from build123d import *

# Parameters (mm, degrees)
SKETCH_R        = 4
PAD_DEPTH       = 6.91
CHAMFER_SIZE    = 0.9674
CHAMFER001_SIZE = 0.9674
GROOVE_ANGLE    = -360


with BuildPart() as part:
    # Sketch → Pad (new body)
    with BuildSketch(Plane.XY):
        Polygon((0, 7), (-6.062178, 3.5), (-6.062178, -3.5), (0, -7), (6.062178, -3.5), (6.062178, 3.5), align=None)
        Circle(SKETCH_R, mode=Mode.SUBTRACT)
    extrude(amount=PAD_DEPTH)

    # Chamfer
    chamfer_edges = [part.edges().sort_by_distance(p)[0] for p in [
        (-4, 0, 6.91),
    ]]
    chamfer(chamfer_edges, length=CHAMFER_SIZE)

    # Chamfer001
    chamfer001_edges = [part.edges().sort_by_distance(p)[0] for p in [
        (-4, 0, 0),
    ]]
    chamfer(chamfer001_edges, length=CHAMFER001_SIZE)

    # Sketch001 → Groove (revolve, symmetric, cut)
    with BuildSketch(Plane.YZ) as groove_sk:
        Polygon((-6.062178, 6.91), (-7, 6.91), (-7, 5.285644), align=None)
        Polygon((-7, 1.624356), (-7, 0), (-6.062178, 0), align=None)
    revolve(axis=Axis((0, 0, 0), (0, 0, 1)), revolution_arc=GROOVE_ANGLE / 2, mode=Mode.SUBTRACT)
    revolve(groove_sk.sketch, axis=Axis((0, 0, 0), (0, 0, -1)), revolution_arc=GROOVE_ANGLE / 2, mode=Mode.SUBTRACT)


solid = part.part
Build history of the part. All positions in model axes, mm. Coordinates: 2 decimals unless noted, no trailing zeros. Write each loop counter-clockwise with the first axis right and the second up, starting at its lowest first coordinate (ties: lowest second). Pieces come first, ordered by that corner, then holes.
(1) Drill centre lines: line 1 (X direction, y = 1.5, z = 5); line 2 (Y direction, x = -1.25, z = 3); line 3 (X direction, y = -3, z = 3.25). Where is each one in solid material? Low to high.
(2) Cut at B-B on z = 6.25. List the corners of the cut face in (x, y), and give its area (3 significant figures).
(3) Pin check, flat tip, straight feed: pin 1 Ø2 at (y, z) = (-5, 3.5) entering from +X. Stop position of the tip, or through.
(4) Cut at A-A on z = 3.5. List the corners of the cut face in (x, y).
Working result:
1. line 1: x = -6.06 to -3.71, 3.71 to 6.06
1. line 2: y = -6.28 to -3.8, 3.8 to 6.28
1. line 3: x = -6.06 to -2.65, 2.65 to 6.06
2. outline: (-6.06, -2.18) arc R6.44 ccw to (-4.92, -4.16) - (-1.14, -6.34) arc R6.44 ccw to (1.14, -6.34) - (4.92, -4.16) arc R6.44 ccw to (6.06, -2.18) - (6.06, 2.18) arc R6.44 ccw to (4.92, 4.16) - (1.14, 6.34) arc R6.44 ccw to (-1.14, 6.34) - (-4.92, 4.16) arc R6.44 ccw to (-6.06, 2.18) - close; hole circle Ø8.61 at (0, 0)
2. area: 65.4 mm2
3. pin 1: stops at x = 5.2
4. outline: (-6.06, -3.5) - (0, -7) - (6.06, -3.5) - (6.06, 3.5) - (0, 7) - (-6.06, 3.5) - close; hole circle Ø8 at (0, 0)
